from build123d import *

# Parameters (mm, degrees)
F0_W     = 116
F0_H     = 116
F1_DEPTH = 50
F2_W     = 110
F2_H     = 110
F3_DEPTH = 45
F4_R     = 5


with BuildPart() as f1:
    # F0 (on Top) → F1 (new body)
    with BuildSketch(Plane.XY):
        Rectangle(F0_W, F0_H)
    extrude(amount=F1_DEPTH)

    # F2 (on Top) → F3 (cut)
    with BuildSketch(Plane.XY):
        Rectangle(F2_W, F2_H)
    extrude(amount=F3_DEPTH, mode=Mode.SUBTRACT)

    # F4
    f4_edges = [f1.edges().sort_by_distance(p)[0] for p in [
        (-58, 58, 25),
        (55, 55, 22.5),
        (-55, -55, 22.5),
        (55, -55, 22.5),
    ]]
    fillet(f4_edges, radius=F4_R)


solid = f1.part
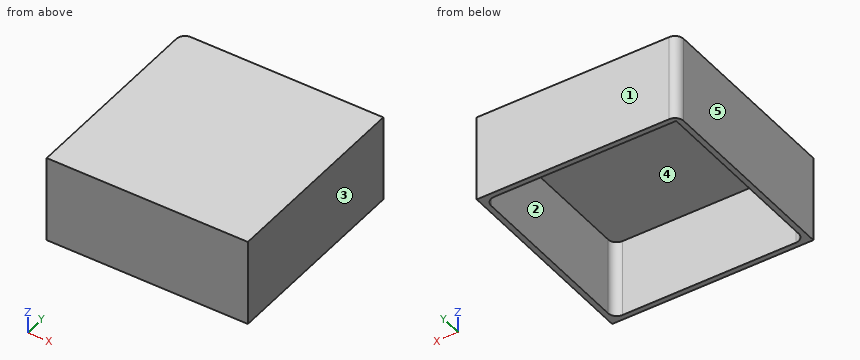
Design review of the part built by this model. Coordinates are the model's own, in mm. Face numbers are marked on the shaded views. A direction names the side the tool comes from. Give positions to 0.01 mm unless a question says otherwise; leave off trailing zeros. Loops run counter-clockwise (first coordinate to the right, second up) from the corner with the lowest first, then second, coordinate; pieces in that order, holes last. Notation, with made-up numbers: M 41.25,-18 L 72.25,-18 A20 ccw 72.25,14 Z; hole C -25,-6.5 d1. An arc over 180 degrees is marked long. One line per question, with ' | ' between items. Start each with the question number.
1. Add section C-C (z = 16). Write out the cut boundary in (x, y).
2. To check wall thickness, follow L1, parallel to Y at x = 0.5, z = 32.5; L2, parallel to Z at x = 0, y = 53. State the ranges of each line that lie inside material, in increasing order.
3. For the marked faces 4 and 5, list the 3-axis set-ups (+Z, -Z, +X, -X, +Y, -Y) from which the entire face can be reached by the end or side of a thin tool; tool diameter is ignored.
4. Add section A-A (y = -8). Write out the cut boundary in (x, z).
5. Insertion check: P1, Ø10, axis at x = 36.5, y = -45.5, coming from the -Z side. The pin has a flat end and moves straight along its axis. Give the tip position at first contact, or say it passes through.
6. The part is to be moulded in two halves that separate along Y. For the marked faces 1, 2 and 3, say which applies: released by +Y, released by -Y, zero draft, split by the parting line, or undercut.
Worked out:
1) outline: M -58,-58 L 58,-58 L 58,58 L -53,58 A5 ccw -58,53 Z; hole M -55,-50 A5 ccw -50,-55 L 50,-55 A5 ccw 55,-50 L 55,50 A5 ccw 50,55 L -55,55 Z
2) L1: y = -58 to -55, 55 to 58 | L2: z = 45 to 50
3) face 4: -Z | face 5: +Z, -Z, -X, +Y, -Y
4) outline: M -58,0 L -55,0 L -55,45 L 55,45 L 55,0 L 58,0 L 58,50 L -58,50 Z
5) P1: stops at z = 45
6) face 1: released by +Y | face 2: undercut | face 3: zero draft
